Verification items for this drawing (mm, ordinates from the low corner). A direction names the side the tool comes from. Coordinates: 2 decimals unless noted, no trailing zeros. Write each loop counter-clockwise with the first axis right and the second up, starting at its lowest first coordinate (ties: lowest second). Pieces come first, ordered by that corner, then holes. Notation, with made-up numbers: (37.25, 60.5) -> (77.25, 60.5) arc R32 ccw to (77.25, 88.5) -> close; hole circle Ø8 at (46.25, 70). An arc over 180 degrees is marked (long way). One line per question, with ' | ' between items.
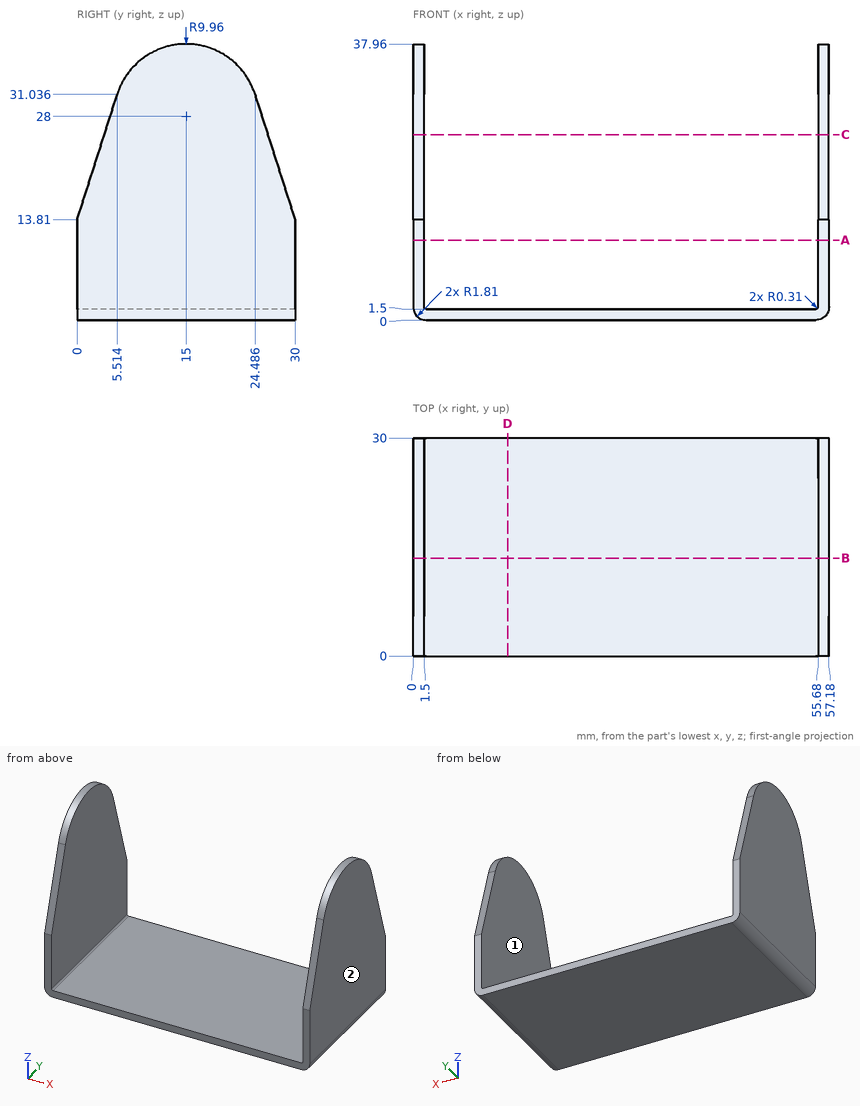
(1) Cross-section at A-A (z = 11). Record the cut outline in (x, y).
Answers below:
outline: (0, 0) -> (1.5, 0) -> (1.5, 30) -> (0, 30) -> close; (55.68, 0) -> (57.18, 0) -> (57.18, 30) -> (55.68, 30) -> close
(2) Cross-section at B-B (y = 13.5). Record the cut outline in (x, z).
Answers below:
outline: (0, 1.81) arc R1.81 ccw to (1.81, 0) -> (55.37, 0) arc R1.81 ccw to (57.18, 1.81) -> (57.18, 37.85) -> (55.68, 37.85) -> (55.68, 1.81) arc R0.31 cw to (55.37, 1.5) -> (1.81, 1.5) arc R0.31 cw to (1.5, 1.81) -> (1.5, 37.85) -> (0, 37.85) -> close
(3) Depth check by flat-ended pin: P1, Ø2, axis at x = 19, y = 20, coming from the +Z side. Enter the tip coordinate at first touch or a pass-through.
Answers below:
P1: stops at z = 1.5
(4) Cross-section at D-D (x = 13). Record the cut outline in (y, z).
Answers below:
outline: (0, 0) -> (30, 0) -> (30, 1.5) -> (0, 1.5) -> close
(5) Material ranges on line 1 (X direction, y = 24, z = 4); line 2 (Z direction, x = 20, y = 14), recorded low to high.
Answers below:
line 1: x = 0 to 1.5, 55.68 to 57.18 | line 2: z = 0 to 1.5
(6) Tool access check on the marked faces 1 and 2. Record the directions out of +Z, -Z, +X, -X, +Y, -Y that give a thin tool (end or side, any length) a straight path to the whole face; none if there is none.
Answers below:
face 1: +Z, +Y, -Y | face 2: +Z, -Z, +X, +Y, -Y
(7) Cross-section at C-C (z = 25.5). Record the cut outline in (x, y).
Answers below:
outline: (0, 3.74) -> (1.5, 3.74) -> (1.5, 26.26) -> (0, 26.26) -> close; (55.68, 3.74) -> (57.18, 3.74) -> (57.18, 26.26) -> (55.68, 26.26) -> close
